Geometry: final body of the model. Coordinates: model frame, mm. A direction names the side the tool comes from. Give positions to 0.01 mm unless a question says otherwise; leave off trailing zeros. Write each loop counter-clockwise with the first axis right and the second up, starting at its lowest first coordinate (ties: lowest second). Pieces come first, ordered by that corner, then holes. Notation, with made-up numbers: (74.25, 44) -> (124.25, 44) arc R21 cw to (124.25, 66) -> close; hole circle Ø10 at (-2, 80.25). An arc over 180 degrees is marked (long way). Use CSV: the item, a comma, the result in double quotes. Start each with the question number.
1) Set-up query: faces 1 (the face through (-77.2, 41.186, 7.3)), 2 (the face through (-74.858, 22, 1)), 3 (the face through (-67, 50.698, 4)). Return all of +Z, -Z, +X, -X, +Y, -Y with unobstructed straight access to the full face (end or side cutting, diameter ignored); none if empty.
2) Draft query along Z for faces 4 (the face through (-72.54, 30.76, 3.22)), 5 (the face through (-65, 31, 0)), 6 (the face through (-78.508, 29.403, 8.417)). Return one class per face: pulls with the +Z half, pulls with the -Z half, needs draft (parallel to the pull), parting line crosses it, or undercut.
3) Section A-A (x = -76). Output: boundary loops of the cut face in (y, z).
4) Section C-C (y = 16.5). Output: boundary loops of the cut face in (x, z), plus the area to 3 significant figures.
5) Material intervals for line 1 (Z direction, x = -66.5, y = 22.5); line 2 (X direction, y = 48, z = 3.25); line 3 (Z direction, x = -72.25, y = 34), sorted ascending. Write a range as [from, to].
6) Section D-D (z = 4.25). Output: boundary loops of the cut face in (x, y).
7) Contact query for flat-ended pins moving along their axis: P1, Ø2, axis at x = -64.5, y = 31.5, coming from the -Z side; P2, Ø10, axis at x = -58, y = 38.5, coming from the +Z side; P3, Ø4.5, axis at x = -74.86, z = 5, coming from the +Y side; P4, Ø2.5, axis at y = 36.5, z = 1, coming from the -X side. Output: stop coordinate, or through.
8) Section B-B (z = 6.25). Output: boundary loops of the cut face in (x, y), plus the area to 3 significant figures.
```python
from build123d import *

# Parameters (mm, degrees)
F0_W     = 20.7803882658
F0_H     = 40.445305407
F1_DEPTH = 5
F2_W     = 9.5119066536
F2_H     = 5
F2_W_2   = 9.1619901359
F2_W_3   = 8.8719539344
F3_ANGLE = 270
F4_R     = 2.9239984628
F5_DEPTH = 100


with BuildPart() as f1:
    # F0 (on Top) → F1 (new body)
    with BuildSketch(Plane.XY):
        with Locations((-64.4678976387, 30.4752923548)):
            Rectangle(F0_W, F0_H)
    extrude(amount=F1_DEPTH)

    # F2 (on face) → F3 (revolve)
    with BuildSketch(Plane(origin=(-74.8580917716, 0, 0), x_dir=(0, -1, 0), z_dir=(-1, 0, 0))):
        with Locations((-45.9419917315, 2.5)):
            Rectangle(F2_W, F2_H)
        with Locations((-29.4675175101, 2.5)):
            Rectangle(F2_W_2, F2_H)
        with Locations((-14.6886166185, 2.5)):
            Rectangle(F2_W_3, F2_H)
    revolve(axis=Axis((-74.8580917716, 28.935774928, 5), (0, 1, 0)), revolution_arc=F3_ANGLE)

    # F4 (on face) → F5 (cut)
    with BuildSketch(Plane(origin=(0, 50.6979450583, 0), x_dir=(-1, 0, 0), z_dir=(0, 1, 0))):
        with Locations((74.8580917716, 5)):
            Circle(F4_R)
    extrude(amount=-F5_DEPTH, mode=Mode.SUBTRACT)


solid = f1.part
```
Answers follow:
1,face 1,"+Z, -X"
1,face 2,"+Z, -Z, -X"
1,face 3,"+Z, -Z, +X, -X, +Y"
2,face 4,"undercut"
2,face 5,"pulls with the -Z half"
2,face 6,"parting line crosses it"
3,outline,"(10.25, 0.13) -> (19.12, 0.13) -> (19.12, 2.31) -> (10.25, 2.31) -> close; (10.25, 7.69) -> (19.12, 7.69) -> (19.12, 9.87) -> (10.25, 9.87) -> close; (24.89, 0.13) -> (34.05, 0.13) -> (34.05, 2.31) -> (24.89, 2.31) -> close; (24.89, 7.69) -> (34.05, 7.69) -> (34.05, 9.87) -> (24.89, 9.87) -> close; (41.19, 0.13) -> (50.7, 0.13) -> (50.7, 2.31) -> (41.19, 2.31) -> close; (41.19, 7.69) -> (50.7, 7.69) -> (50.7, 9.87) -> (41.19, 9.87) -> close"
4,outline,"(-74.86, 0) -> (-54.08, 0) -> (-54.08, 5) -> (-69.86, 5) arc R5 ccw (long way) to start; hole circle Ø5.85 at (-74.86, 5)"
4,area,"136 mm^2"
5,line 1,"z = [0, 5]"
5,line 2,"x = [-79.54, -77.2], [-72.52, -54.08]"
5,line 3,"z = [0, 3.68], [6.32, 9.27]"
6,outline,"(-79.8, 10.25) -> (-77.68, 10.25) -> (-77.68, 19.12) -> (-79.8, 19.12) -> close; (-79.8, 24.89) -> (-77.68, 24.89) -> (-77.68, 34.05) -> (-79.8, 34.05) -> close; (-79.8, 41.19) -> (-77.68, 41.19) -> (-77.68, 50.7) -> (-79.8, 50.7) -> close; (-72.03, 10.25) -> (-54.08, 10.25) -> (-54.08, 50.7) -> (-72.03, 50.7) -> close"
7,P1,"stops at z = 0"
7,P2,"stops at z = 5"
7,P3,"passes through"
7,P4,"stops at x = -74.86"
8,outline,"(-79.7, 10.25) -> (-77.5, 10.25) -> (-77.5, 19.12) -> (-79.7, 19.12) -> close; (-79.7, 24.89) -> (-77.5, 24.89) -> (-77.5, 34.05) -> (-79.7, 34.05) -> close; (-79.7, 41.19) -> (-77.5, 41.19) -> (-77.5, 50.7) -> (-79.7, 50.7) -> close; (-72.21, 10.25) -> (-70.02, 10.25) -> (-70.02, 19.12) -> (-72.21, 19.12) -> close; (-72.21, 24.89) -> (-70.02, 24.89) -> (-70.02, 34.05) -> (-72.21, 34.05) -> close; (-72.21, 41.19) -> (-70.02, 41.19) -> (-70.02, 50.7) -> (-72.21, 50.7) -> close"
8,area,"121 mm^2"
